For this review, take the finished solid that the model builds, in its own axes (mm). A direction names the side the tool comes from. Give positions to 0.01 mm unless a question says otherwise; leave off trailing zeros. Loops run counter-clockwise (first coordinate to the right, second up) from the corner with the lowest first, then second, coordinate; pieces in that order, holes last.
```python
from build123d import *

# Parameters (mm, degrees)
SKETCH1_R                = 20
BOSS_EXTRUDE1_DEPTH      = 8
BOSS_EXTRUDE3_START      = 22
BOSS_EXTRUDE3_DEPTH      = 4
CIRPATTERN1_COUNT        = 3
CIRPATTERN1_START        = 22
CIRPATTERN1_COPY_1_DEPTH = 4
CIRPATTERN1_COPY_2_DEPTH = 4
SKETCH4_R                = 2.1
CUT_EXTRUDE1_DEPTH       = 83.250631167
CIRPATTERN2_COUNT        = 6
FILLET2_R                = 2
FILLET4_R                = 1.5
FILLET5_R                = 2


with BuildPart() as part:
    # Sketch1 → Boss-Extrude1 (new body)
    with BuildSketch(Plane.XY):
        Polygon((49.074772881, -5), (20.207259422, 45), (-20.207259422, 45), (-49.074772881, -5), (-28.867513459, -40), (28.867513459, -40), align=None)
        Circle(SKETCH1_R, mode=Mode.SUBTRACT)
    extrude(amount=BOSS_EXTRUDE1_DEPTH)

    # Sketch3 → Boss-Extrude3 (add)
    with BuildSketch(Plane(origin=(0, 0, 0), x_dir=(0, 0, -1), z_dir=(1, 0, 0)).offset(BOSS_EXTRUDE3_START)):
        with BuildLine():
            Line((0, -40), (0, -55))
            Line((0, -55), (-4, -55))
            ThreePointArc((-4, -55), (-6.828427125, -53.828427125), (-8, -51))
            Line((-8, -51), (-8, -40))
            Line((-8, -40), (0, -40))
        make_face()
        Polygon((-4, -48.267949192), (-5.5, -49.133974596), (-5.5, -50.866025404), (-4, -51.732050808), (-2.5, -50.866025404), (-2.5, -49.133974596), align=None, mode=Mode.SUBTRACT)
    boss_extrude3 = extrude(amount=BOSS_EXTRUDE3_DEPTH)

    # Mirror1: Boss-Extrude3 across plane
    add(boss_extrude3.mirror(Plane(origin=(0, 0, 0), x_dir=(0, 0, 1), z_dir=(1, 0, 0))))

    # CirPattern1: Boss-Extrude3 ×3 about axis
    cirpattern1_axis = Axis((0, 0, 0), (0, 0, 1))
    for i in range(1, CIRPATTERN1_COUNT):
        add(boss_extrude3.rotate(cirpattern1_axis, i * 360 / CIRPATTERN1_COUNT))

    # CirPattern1 copy 1 sketch → CirPattern1 copy 1 (add)
    with BuildSketch(Plane(origin=(0, 0, 0), x_dir=(0, 0, -1), z_dir=(0.4999999999999998, -0.8660254037844387, 0)).offset(CIRPATTERN1_START)):
        with BuildLine():
            Line((0, 40), (0, 55))
            Line((0, 55), (-4, 55))
            ThreePointArc((-4, 55), (-6.828427125, 53.828427125), (-8, 51))
            Line((-8, 51), (-8, 40))
            Line((-8, 40), (0, 40))
        make_face()
        Polygon((-4, 48.267949192), (-5.5, 49.133974596), (-5.5, 50.866025404), (-4, 51.732050808), (-2.5, 50.866025404), (-2.5, 49.133974596), align=None, mode=Mode.SUBTRACT)
    extrude(amount=CIRPATTERN1_COPY_1_DEPTH)

    # CirPattern1 copy 2 sketch → CirPattern1 copy 2 (add)
    with BuildSketch(Plane(origin=(0, 0, 0), x_dir=(0, 0, -1), z_dir=(0.5000000000000004, 0.8660254037844384, 0)).offset(CIRPATTERN1_START)):
        with BuildLine():
            Line((0, 40), (0, 55))
            Line((0, 55), (-4, 55))
            ThreePointArc((-4, 55), (-6.828427125, 53.828427125), (-8, 51))
            Line((-8, 51), (-8, 40))
            Line((-8, 40), (0, 40))
        make_face()
        Polygon((-4, 48.267949192), (-5.5, 49.133974596), (-5.5, 50.866025404), (-4, 51.732050808), (-2.5, 50.866025404), (-2.5, 49.133974596), align=None, mode=Mode.SUBTRACT)
    extrude(amount=CIRPATTERN1_COPY_2_DEPTH)

    # Sketch4 → Cut-Extrude1 (cut, through all)
    with BuildSketch(Plane.XY.offset(8)):
        with Locations((0, 25)):
            Circle(SKETCH4_R)
    cut_extrude1 = extrude(amount=-CUT_EXTRUDE1_DEPTH, mode=Mode.SUBTRACT)

    # CirPattern2: Cut-Extrude1 ×6 about axis
    cirpattern2_axis = Axis((0, 0, 0), (0, 0, 1))
    for i in range(1, CIRPATTERN2_COUNT):
        add(cut_extrude1.rotate(cirpattern2_axis, i * 360 / CIRPATTERN2_COUNT), mode=Mode.SUBTRACT)

    # Fillet2
    fillet2_edges = [part.edges().sort_by_distance(p)[0] for p in [
        (-26, -40, 4),
        (-22, -40, 4),
        (26, -40, 4),
        (22, -40, 4),
        (-47.641016151, -2.516660498, 4),
        (-23.641016151, 39.052558883, 4),
        (-45.641016151, 0.947441117, 4),
        (-21.641016151, 42.516660498, 4),
        (23.641016151, 39.052558883, 4),
        (21.641016151, 42.516660498, 4),
        (45.641016151, 0.947441117, 4),
        (47.641016151, -2.516660498, 4),
    ]]
    fillet(fillet2_edges, radius=FILLET2_R)

    # Fillet4
    # the kernel refuses this fillet: 1.5 mm, written as the material it takes off along each edge
    with BuildSketch(Plane(origin=(36.631397208, 46.552558883, -3.75), x_dir=(-0.8660254037844387, -0.5, -1.7763568394002503e-15), z_dir=(0, 0, 1)), Plane(origin=(34.631397208, 50.016660498, -3.75), x_dir=(0.5, -0.8660254037844387, 0), z_dir=(0, 0, 1)), Plane(origin=(58.631397208, 8.447441117, -3.75), x_dir=(0.4999999999999998, -0.8660254037844389, 0), z_dir=(0, 0, 1)), Plane(origin=(60.631397208, 4.983339502, -3.75), x_dir=(-0.866025403784439, -0.4999999999999993, -1.7763568394002505e-15), z_dir=(0, 0, 1)), Plane(origin=(-36.631397208, 46.552558883, -3.75), x_dir=(0.5, 0.8660254037844387, 0), z_dir=(0, 0, 1)), Plane(origin=(-34.631397208, 50.016660498, -3.75), x_dir=(0.8660254037844398, -0.49999999999999795, -1.7763568394002505e-15), z_dir=(0, 0, 1))) as fillet4_piece_1:
        with BuildLine():
            CenterArc((FILLET4_R, -FILLET4_R), FILLET4_R, 90, 90)
            Line((0, -FILLET4_R), (0, 0))
            Line((0, 0), (FILLET4_R, 0))
        make_face()
    extrude(amount=11.5, mode=Mode.SUBTRACT)
    with BuildSketch(Plane(origin=(-60.631397208, 4.983339502, -3.75), x_dir=(0.8660254037844379, -0.5000000000000011, -1.7763568394002503e-15), z_dir=(0, 0, 1)), Plane(origin=(-58.631397208, 8.447441117, -3.75), x_dir=(-0.5, -0.8660254037844387, 0), z_dir=(0, 0, 1)), Plane(origin=(26, -55, -3.75), x_dir=(0, 1, 0), z_dir=(0, 0, 1)), Plane(origin=(22, -55, -3.75), x_dir=(1, 0, 0), z_dir=(0, 0, 1)), Plane(origin=(-26, -55, -3.75), x_dir=(1, 0, 0), z_dir=(0, 0, 1)), Plane(origin=(-22, -55, -3.75), x_dir=(0, 1, 0), z_dir=(0, 0, 1))) as fillet4_piece_2:
        with BuildLine():
            CenterArc((FILLET4_R, FILLET4_R), FILLET4_R, 180, 90)
            Line((0, FILLET4_R), (0, 0))
            Line((0, 0), (FILLET4_R, 0))
        make_face()
    extrude(amount=11.5, mode=Mode.SUBTRACT)

    # Fillet5
    fillet5_edges = [part.edges().sort_by_distance(p)[0] for p in [
        (20.207259422, 45, 4),
        (-20.207259422, 45, 4),
        (-49.074772881, -5, 4),
        (-28.867513459, -40, 4),
        (49.074772881, -5, 4),
        (28.867513459, -40, 4),
    ]]
    fillet(fillet5_edges, radius=FILLET5_R)


solid = part.part
```
Q1. Consider section C-C on y = -12.5. Give the boundary of the cut face in (x, z), plus the area to 3 significant figures.
Answers:
outline: (-44.74, 0) - (-23.75, 0) - (-23.75, 8) - (-44.74, 8) - close; (-19.55, 0) - (-15.61, 0) - (-15.61, 8) - (-19.55, 8) - close; (15.61, 0) - (19.55, 0) - (19.55, 8) - (15.61, 8) - close; (23.75, 0) - (44.74, 0) - (44.74, 8) - (23.75, 8) - close
area: 399 mm2
Q2. Consider section A-A on x = 0. Give the boundary of the cut face in (y, z), plus the area to 3 significant figures.
Answers:
outline: (-40, 0) - (-27.1, 0) - (-27.1, 8) - (-40, 8) - close; (-22.9, 0) - (-20, 0) - (-20, 8) - (-22.9, 8) - close; (20, 0) - (22.9, 0) - (22.9, 8) - (20, 8) - close; (27.1, 0) - (45, 0) - (45, 8) - (27.1, 8) - close
area: 293 mm2
Q3. Consider section B-B on y = 0. Give the boundary of the cut face in (x, z), plus the area to 3 significant figures.
Answers:
outline: (-52, 0) - (-20, 0) - (-20, 8) - (-52, 8) - close; (20, 0) - (52, 0) - (52, 8) - (20, 8) - close
area: 512 mm2
Q4. Mouldability with a two-part tool opening along Y and no side actions: class faces 1 (the cylindrical face through (-34.2, 47.43, 7.25)), 2 (the flat face through (0, -40, 4)), 3 (the flat face through (30.283, 42.887, 3.944)) as +Y half, -Y half, draft (parallel to the pull), parting line (faces both ways), or undercut.
Answers:
face 1: +Y half
face 2: -Y half
face 3: undercut
Q5. Consider section D-D on x = 13. Give the boundary of the cut face in (y, z).
Answers:
outline: (-40, 0) - (-15.2, 0) - (-15.2, 8) - (-40, 8) - close; (15.2, 0) - (45, 0) - (45, 8) - (15.2, 8) - close
Q6. For pin 1 Ø4 at (x, z) = (9, 2.5) entering from +Y; pin 2 Ø1.5 at (x, z) = (-32.5, 2.5) entering from -Y; pin 3 Ø4 at (x, z) = (35, 1.5) entering from -Y, all flat-tipped, find the tip position at first contact; note any pin that passes through.
Answers:
pin 1: stops at y = 45
pin 2: stops at y = -35.01
pin 3: stops at y = -32.84
Q7. For probe 1 along Y at (x, z) = (0, 1.5); probe 2 along X at (y, z) = (-13, 7.5); probe 3 along X at (y, z) = (-4, 6.5), list the stretches that pass through material, from the lowest coordinate up.
Answers:
probe 1: y = -40 to -27.1, -22.9 to -20, 20 to 22.9, 27.1 to 45
probe 2: x = -44.46 to -23.69, -19.61 to -15.2, 15.2 to 19.61, 23.69 to 44.46
probe 3: x = -48.52 to -19.6, 19.6 to 48.52
Q8. Machinability: for faces 4 (the flat face through (55, 4, 5.5)), 5 (the flat face through (-26, -48, 4)), 6 (the flat face through (22, -48, 4)), which of the approach directions +Z, -Z, +X, -X, +Y, -Y give a long, thin tool a straight path to every point of the face, cutting with its end or side? Answer none if there is none.
Answers:
face 4: none
face 5: +Z, -Z, -X, -Y
face 6: +Z, -Z, -Y
